from build123d import *

# Parameters (mm, degrees)
F0_W     = 390.525
F0_H     = 390.525
F0_W_2   = 381
F0_H_2   = 381
F1_DEPTH = 625.475
F2_DEPTH = 4.6355
F4_W     = 381
F4_H     = 381
F5_DEPTH = 4.6355


with BuildPart() as f1:
    # F0 (on Top) → F1 (new body)
    with BuildSketch(Plane.XY):
        with Locations((195.2625, 195.2625)):
            Rectangle(F0_W, F0_H)
        with Locations((195.2625, 195.2625)):
            Rectangle(F0_W_2, F0_H_2, mode=Mode.SUBTRACT)
    extrude(amount=F1_DEPTH)

    # F0 (on Top) → F2 (join)
    with BuildSketch(Plane.XY):
        with Locations((195.2625, 195.2625)):
            Rectangle(F0_W_2, F0_H_2)
    extrude(amount=F2_DEPTH)

    # F4 (on plane+point) → F5 (join)
    with BuildSketch(Plane.XY.offset(625.475)):
        Polygon((-190.5, 0), (0, 0), (0, -165.1), (390.525, -165.1), (390.525, 0), (581.025, 0), (581.025, 390.525), (390.525, 390.525), (390.525, 555.625), (0, 555.625), (0, 390.525), (-190.5, 390.525), align=None)
        with Locations((195.2625, 195.2625)):
            Rectangle(F4_W, F4_H, mode=Mode.SUBTRACT)
    extrude(amount=F5_DEPTH)


solid = f1.part
Source: CAD feature listing. Evaluate the final solid. Frame: model axes, mm. A direction names the side the tool comes from. Round coordinates to 2 decimals unless told otherwise and drop trailing zeros. Write each loop counter-clockwise with the first axis right and the second up, starting at its lowest first coordinate (ties: lowest second). Pieces come first, ordered by that corner, then holes. Notation, with made-up numbers: M 78,-15.5 L 109,-15.5 A21 ccw 109,23.5 Z; hole C 1.25,75.25 d2. An arc over 180 degrees is marked long. One line per item, written item: value. Start each with the question number.
Item 1: Section query A-A (z = 43). Return the cut outline in (x, y) (1 decimal), plus the area to 3 significant figures.
Item 2: Pin query (flat end, axial travel): pin 1 (6 mm diameter, centred on x = 21.5, z = 145, fed in from +Y) (3 decimals); pin 2 (1.5 mm diameter, centred on x = -34, y = 350, fed in from -Z) (3 decimals); pin 3 (1 mm diameter, centred on x = 333, y = 33.5, fed in from -Z); pin 4 (3.5 mm diameter, centred on x = 446, z = 629, fed in from -Y). Return the tip coordinate at first contact, or that it passes through.
Item 3: Section query B-B (x = 111.5). Return the cut outline in (y, z) (1 decimal).
Item 4: Section query C-C (y = 27.5). Return the cut outline in (x, z) (1 decimal).
Item 5: Section query D-D (x = -58.5). Return the cut outline in (y, z) (1 decimal), plus the area to 3 significant figures.
Item 6: Mould query, pull axis Y, two halves, no side actions, for faces 6 (the flat face through (193, 390.525, 308)), 7 (the flat face through (193, 0, 308)), 8 (the flat face through (193, 474, 625.475)), 9 (the flat face through (193, 385.762, 313)). Classes: pulls with the +Y half, pulls with the -Y half, needs draft (parallel to the pull), parting line crosses it, or undercut.
Item 7: Ray query, L1, parallel to Y at x = 6.5, z = 51.5 (1 decimal); L2, parallel to Z at x = -84, y = 28 (1 decimal). Return the intervals inside material, ascending. Write a range as from..to.
Item 8: Set-up query: faces 1 (the flat face through (385.762, 193, 313)), 2 (the flat face through (190, -40, 630.11)), 3 (the flat face through (193, -81, 625.475)), 4 (the flat face through (0, 193, 308)), 5 (the flat face through (484, 198, 625.475)). Return all of +Z, -Z, +X, -X, +Y, -Y with unobstructed straight access to the full face (end or side cutting, diameter ignored); none if empty.
Result set:
1. outline: M 0,0 L 390.5,0 L 390.5,390.5 L 0,390.5 Z; hole M 4.8,4.8 L 385.8,4.8 L 385.8,385.8 L 4.8,385.8 Z
1. area: 7,350 mm²
2. pin 1: stops at y = 390.525
2. pin 2: stops at z = 625.475
2. pin 3: stops at z = 0
2. pin 4: stops at y = 0
3. outline: M -165.1,625.5 L 0,625.5 L 0,0 L 390.5,0 L 390.5,625.5 L 555.6,625.5 L 555.6,630.1 L 385.8,630.1 L 385.8,4.6 L 4.8,4.6 L 4.8,630.1 L -165.1,630.1 Z
4. outline: M -190.5,625.5 L 0,625.5 L 0,0 L 390.5,0 L 390.5,625.5 L 581,625.5 L 581,630.1 L 385.8,630.1 L 385.8,4.6 L 4.8,4.6 L 4.8,630.1 L -190.5,630.1 Z
5. outline: M 0,625.5 L 390.5,625.5 L 390.5,630.1 L 0,630.1 Z
5. area: 1,810 mm²
6. face 6: pulls with the +Y half
6. face 7: pulls with the -Y half
6. face 8: needs draft
6. face 9: undercut
7. L1: y = 0..4.8, 385.8..390.5
7. L2: z = 625.5..630.1
8. face 1: +Z
8. face 2: +Z, +X, -X, +Y, -Y
8. face 3: -Z, +X, -X, -Y
8. face 4: -Z, -X, +Y, -Y
8. face 5: -Z, +X, +Y, -Y
